from build123d import *

# Parameters (mm, degrees)
F1_DEPTH  = 12.6
F2_W      = 10.3
F2_H      = 10.3
F3_DEPTH  = 6
F4_W      = 10.3
F4_H      = 10.3
F5_DEPTH  = 6
F6_R      = 4.2
F7_DEPTH  = 3.5
F8_R      = 4.2
F9_DEPTH  = 3.5
F11_DEPTH = 6
F13_DEPTH = 3.5


with BuildPart() as f1:
    # F0 (on Top) → F1 (new body)
    with BuildSketch(Plane.XY):
        with BuildLine():
            Line((0, -12.6), (0, 0))
            Line((0, 0), (-21.9674337148, 0))
            ThreePointArc((-21.9674337148, 0), (-28.8956369451, -4), (-28.8956369451, -12))
            Line((-28.8956369451, -12), (-17.9119200877, -31.024355653))
            Line((-17.9119200877, -31.024355653), (-7, -24.724355653))
            Line((-7, -24.724355653), (-14, -12.6))
            Line((-14, -12.6), (0, -12.6))
        make_face()
    extrude(amount=F1_DEPTH)

    # F2 (on face) → F3 (cut)
    with BuildSketch(Plane(origin=(8.9559600438, -15.5121778265, 0), x_dir=(0.8660254038, 0.5, 0), z_dir=(0.5, -0.8660254038, 0))):
        with Locations((-24.724355653, 6.3)):
            Rectangle(F2_W, F2_H)
    extrude(amount=-F3_DEPTH, mode=Mode.SUBTRACT)

    # F4 (on face) → F5 (cut)
    with BuildSketch(Plane.YZ):
        with Locations((-6.3, 6.3)):
            Rectangle(F4_W, F4_H)
    extrude(amount=-F5_DEPTH, mode=Mode.SUBTRACT)

    # F6 (on face) → F7 (cut)
    with BuildSketch(Plane.YZ.offset(-6)):
        with Locations((-6.3, 6.3)):
            Circle(F6_R)
    extrude(amount=-F7_DEPTH, mode=Mode.SUBTRACT)

    # F8 (on face) → F9 (cut)
    with BuildSketch(Plane(origin=(5.9559600438, -10.3160254038, 0), x_dir=(0.8660254038, 0.5, 0), z_dir=(0.5, -0.8660254038, 0))):
        with Locations((-24.724355653, 6.3)):
            Circle(F8_R)
    extrude(amount=-F9_DEPTH, mode=Mode.SUBTRACT)

    # F10 (on face) → F11 (cut)
    with BuildSketch(Plane.XY.offset(12.6)):
        Polygon((-19.5194863729, -15.3600308295), (-14.3694863729, -6.4399691705), (-23.2895480318, -1.2899691705), (-25.8645480318, -5.75), (-28.4395480318, -10.2100308295), align=None)
    extrude(amount=-F11_DEPTH, mode=Mode.SUBTRACT)

    # F12 (on face) → F13 (cut)
    with BuildSketch(Plane.XY.offset(6.6)):
        with BuildLine():
            ThreePointArc((-17.2045172024, -8.325), (-17.7672105065, -6.225), (-19.3045172024, -4.6876933041))
            Line((-19.3045172024, -4.6876933041), (-21.4045172024, -8.325))
            Line((-21.4045172024, -8.325), (-23.5045172024, -11.9623066959))
            ThreePointArc((-23.5045172024, -11.9623066959), (-19.3045172024, -11.9623066959), (-17.2045172024, -8.325))
        make_face()
        with BuildLine():
            Line((-21.4045172024, -8.325), (-19.3045172024, -4.6876933041))
            ThreePointArc((-19.3045172024, -4.6876933041), (-25.0418238983, -6.225), (-23.5045172024, -11.9623066959))
            Line((-23.5045172024, -11.9623066959), (-21.4045172024, -8.325))
        make_face()
    extrude(amount=-F13_DEPTH, mode=Mode.SUBTRACT)


solid = f1.part
Source: CAD feature listing. Evaluate the final solid. Frame: model axes, mm. A direction names the side the tool comes from. Give positions to 0.01 mm unless a question says otherwise; leave off trailing zeros. Order: outer loops, then holes, each group sorted by start corner. A loop starts at its lowest first (then second) coordinate and runs counter-clockwise, first axis right, second up. Notation, with made-up numbers: (10, -7.5) -> (67, -7.5) arc R16 ccw to (67, 23.5) -> close; hole circle Ø6 at (56, 5). An arc over 180 degrees is marked (long way). Use a Markdown table: item, result.
1) Ray query, line 1 along Z through (x, y) = (-14.5, -25.5); line 2 along Y through (x, z) = (-18.5, 10.5); line 3 along Z through (x, y) = (-7.6, -6.3). Return the intervals inside material, ascending. Write a range as [from, to].
Answer list:
| item | result |
|---|---|
| line 1 | [0, 1.15], [11.45, 12.6] |
| line 2 | [-30.01, -27.71], [-24.44, -13.59], [-4.06, 0] |
| line 3 | [0, 2.1], [10.5, 12.6] |
2) Reachability of faces 1 (the flat face through (-3, -6, 1.15)), 2 (the flat face through (-10.45, -18.75, 6.21)), 3 (the flat face through (-17, -11, 10)) from +Z, -Z, +X, -X, +Y, -Y: full face, straight path, thin tool, end or side. Return the list, or none.
Answer list:
| item | result |
|---|---|
| face 1 | +X |
| face 2 | +Z, -Z, +X |
| face 3 | +Z |
3) Mould query, pull axis Z, two halves, no side actions, for faces 4 (the flat face through (-3, -6, 11.45)), 5 (the flat face through (0, -0.8, 6.2)), 6 (the flat face through (-15, -12, 0)). Classes: +Z half, -Z half, draft (parallel to the pull), parting line (faces both ways), or undercut.
Answer list:
| item | result |
|---|---|
| face 4 | undercut |
| face 5 | draft |
| face 6 | -Z half |
4) Contact query for flat-ended pins moving along their axis: P1, Ø1.5, axis at x = -16, z = 6.5, coming from the -Y side; P2, Ø1, axis at x = -9, z = 4, coming from the -Y side; P3, Ø1, axis at y = -15.5, z = 8, coming from the +X side. Output: stop coordinate, or through.
Answer list:
| item | result |
|---|---|
| P1 | y = -19.38 |
| P2 | y = -24.43 |
| P3 | x = -12.04 |
5) Section query A-A, the plane x = -4.25. Return the cut outline in (y, z), then the cut area to 3 significant figures.
Answer list:
| item | result |
|---|---|
| outline | (-12.6, 0) -> (0, 0) -> (0, 12.6) -> (-12.6, 12.6) -> close; hole (-11.45, 1.15) -> (-1.15, 1.15) -> (-1.15, 11.45) -> (-11.45, 11.45) -> close |
| area | 52.7 mm² |
6) Section query C-C, the plane x = -8.5. Return the cut outline in (y, z).
Answer list:
| item | result |
|---|---|
| outline | (-25.59, 0) -> (-22.13, 0) -> (-22.13, 12.6) -> (-25.59, 12.6) -> (-25.59, 11.45) -> (-24.43, 11.45) -> (-24.43, 1.15) -> (-25.59, 1.15) -> close; (-12.6, 0) -> (0, 0) -> (0, 12.6) -> (-12.6, 12.6) -> close; hole circle Ø8.4 at (-6.3, 6.3) |
7) Section query D-D, the plane x = -27. Return the cut outline in (y, z).
Answer list:
| item | result |
|---|---|
| outline | (-15.28, 0) -> (-1.78, 0) -> (-1.78, 12.6) -> (-7.72, 12.6) -> (-7.72, 6.6) -> (-11.04, 6.6) -> (-11.04, 12.6) -> (-15.28, 12.6) -> close |
8) Section query B-B, the plane z = 11. Return the cut outline in (x, y), then the cut area to 3 significant figures.
Answer list:
| item | result |
|---|---|
| outline | (-28.9, -12) -> (-17.91, -31.02) -> (-16.92, -30.45) -> (-19.92, -25.25) -> (-11, -20.1) -> (-8, -25.3) -> (-7, -24.72) -> (-14, -12.6) -> (0, -12.6) -> (0, -11.45) -> (-6, -11.45) -> (-6, -1.15) -> (0, -1.15) -> (0, 0) -> (-21.97, 0) arc R8 ccw to start; hole (-28.44, -10.21) -> (-19.52, -15.36) -> (-14.37, -6.44) -> (-23.29, -1.29) -> close |
| area | 354 mm² |
